```python
from build123d import *

# Parameters (mm, degrees)
F0_W      = 50.8
F0_H      = 50.8
F1_DEPTH  = 25.4
F3_D      = 12.7
F3_DEPTH  = 2.54
F3_TIP    = 3.8154649308
F5_D      = 12.7
F5_DEPTH  = 2.54
F5_TIP    = 3.8154649308
F7_D      = 12.7
F7_DEPTH  = 2.54
F7_TIP    = 3.8154649308
F9_D      = 12.7
F9_DEPTH  = 2.54
F9_TIP    = 3.8154649308
F12_D     = 12.7
F12_DEPTH = 2.54
F12_TIP   = 3.8154649308
F14_D     = 12.7
F14_DEPTH = 2.54
F14_TIP   = 3.8154649308
F16_D     = 12.7
F16_DEPTH = 2.54
F16_TIP   = 3.8154649308
F17_R     = 2.54


with BuildPart() as f1:
    # F0 (on Front) → F1 (new body, symmetric)
    with BuildSketch(Plane.XZ):
        Rectangle(F0_W, F0_H)
    extrude(amount=F1_DEPTH, both=True)

    # F3
    with Locations(Plane.XZ.offset(25.4)):
        with Locations((0, 0)):
            Hole(F3_D / 2, depth=F3_DEPTH)
            with Locations((0, 0, -(F3_DEPTH + F3_TIP / 2))):  # 118° drill point
                Cone(0, F3_D / 2, F3_TIP, mode=Mode.SUBTRACT)

    # F5
    with Locations(Plane(origin=(0, 25.4, 0), x_dir=(-1, 0, 0), z_dir=(0, 1, 0))):
        with Locations((-15.24, 15.24), (0, 0), (15.24, -15.24)):
            Hole(F5_D / 2, depth=F5_DEPTH)
            with Locations((0, 0, -(F5_DEPTH + F5_TIP / 2))):  # 118° drill point
                Cone(0, F5_D / 2, F5_TIP, mode=Mode.SUBTRACT)

    # F7
    with Locations(Plane.XY.offset(25.4)):
        with Locations((-15.24, 15.24), (15.24, -15.24)):
            Hole(F7_D / 2, depth=F7_DEPTH)
            with Locations((0, 0, -(F7_DEPTH + F7_TIP / 2))):  # 118° drill point
                Cone(0, F7_D / 2, F7_TIP, mode=Mode.SUBTRACT)

    # F9
    with Locations(Plane(origin=(0, 0, -25.4), x_dir=(1, 0, 0), z_dir=(0, 0, -1))):
        with Locations((-15.24, 15.24), (15.24, 15.24), (15.24, -15.24), (-15.24, -15.24)):
            Hole(F9_D / 2, depth=F9_DEPTH)
            with Locations((0, 0, -(F9_DEPTH + F9_TIP / 2))):  # 118° drill point
                Cone(0, F9_D / 2, F9_TIP, mode=Mode.SUBTRACT)

    # F12
    with Locations(Plane(origin=(0, 25.4, 0), x_dir=(-1, 0, 0), z_dir=(0, 1, 0))):
        with Locations((15.24, 15.24), (-15.24, -15.24)):
            Hole(F12_D / 2, depth=F12_DEPTH)
            with Locations((0, 0, -(F12_DEPTH + F12_TIP / 2))):  # 118° drill point
                Cone(0, F12_D / 2, F12_TIP, mode=Mode.SUBTRACT)

    # F14
    with Locations(Plane.YZ.offset(25.4)):
        with Locations((-15.24, 15.24), (0, 0), (15.24, -15.24)):
            Hole(F14_D / 2, depth=F14_DEPTH)
            with Locations((0, 0, -(F14_DEPTH + F14_TIP / 2))):  # 118° drill point
                Cone(0, F14_D / 2, F14_TIP, mode=Mode.SUBTRACT)

    # F16
    with Locations(Plane(origin=(-25.4, 0, 0), x_dir=(0, -1, 0), z_dir=(-1, 0, 0))):
        with Locations((-15.24, 15.24), (-15.24, 0), (-15.24, -15.24), (15.24, -15.24), (15.24, 0), (15.24, 15.24)):
            Hole(F16_D / 2, depth=F16_DEPTH)
            with Locations((0, 0, -(F16_DEPTH + F16_TIP / 2))):  # 118° drill point
                Cone(0, F16_D / 2, F16_TIP, mode=Mode.SUBTRACT)

    # F17
    f17_edges = [f1.edges().sort_by_distance(p)[0] for p in [
        (-25.4, 0, 25.4),
        (0, 25.4, 25.4),
        (-25.4, 25.4, 0),
        (0, -25.4, 25.4),
        (25.4, 0, 25.4),
        (25.4, 25.4, 0),
        (25.4, -25.4, 0),
        (25.4, 0, -25.4),
        (0, 25.4, -25.4),
        (-25.4, 0, -25.4),
        (-25.4, -25.4, 0),
        (0, -25.4, -25.4),
    ]]
    fillet(f17_edges, radius=F17_R)


solid = f1.part
```
The model under review builds one solid part; all positions refer to its coordinate system, in mm. A direction names the side the tool comes from. Round coordinates to 2 decimals unless told otherwise and drop trailing zeros.
1) Clearance check with flat-ended pins moving along their axes: P1, Ø16.5, axis at y = -15.24, z = -15.24, coming from the -X side; P2, Ø7.5, axis at x = 15.24, y = 15.24, coming from the -Z side; P3, Ø11.5, axis at x = -15.24, y = 15.24, coming from the -Z side; P4, Ø11.5, axis at y = 15.24, z = 0, coming from the -X side. State where each tip first meets the part, or that it passes through.
Values follow:
P1: stops at x = -25.4
P2: stops at z = -21.3
P3: stops at z = -22.5
P4: stops at x = -22.5
2) The part is to be moulded in two halves that separate along Z. For faces 1 (the face through (-14.647, 16.17, 19.707)), 2 (the face through (24.11, 1.38, -6.2)), 3 (the face through (21.584, -15.519, -24.112)), say which applies: pulls with the +Z half, pulls with the -Z half, needs draft (parallel to the pull), parting line crosses it, or undercut.
Values follow:
face 1: pulls with the +Z half
face 2: undercut
face 3: needs draft
3) Tool access review of faces 4 (the face through (21.584, -14.961, 24.112)), 5 (the face through (-21.584, 24.112, -14.961)), 6 (the face through (24.112, 21.584, -14.961)): name each direction out of +Z, -Z, +X, -X, +Y, -Y from which nothing blocks a thin tool from reaching the whole face with its end or side.
Values follow:
face 4: +Z
face 5: +Y
face 6: +X
4) Wall thickness on line 1 along X through (y, z) = (23, 15); line 2 along Y through (x, z) = (15.24, -24.8); line 3 along Z through (x, y) = (-15.24, 24.6): over which ranges is each line inside the solid? List them lowest first.
Values follow:
line 1: x = -25.4 to -21.59, -8.89 to 8.89, 21.59 to 25.4
line 2: y = -24.5 to -21.59, -8.89 to 8.89, 21.59 to 24.5
line 3: z = -24.71 to -21.59, -8.89 to 8.89, 21.59 to 24.71
